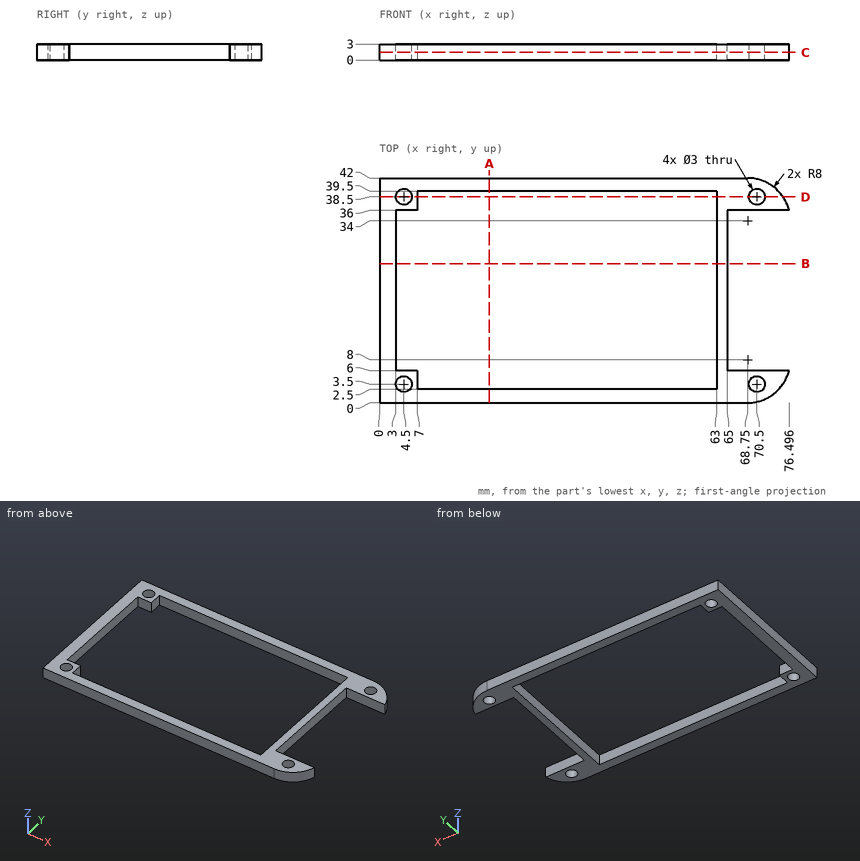
Could you check a few things on this drawing? It's one solid part, dimensions in mm from its lowest x, y, z. Round coordinates to 2 decimals unless told otherwise and drop trailing zeros. Order: outer loops, then holes, each group sorted by start corner. A loop starts at its lowest first (then second) coordinate and runs counter-clockwise, first axis right, second up. Notation, with made-up numbers: M -13,29 L -2,29 A29 ccw -2,56 Z; hole C -3,31 d9. An arc over 180 degrees is marked long. Return JSON: item names as keys, results as strings. Group by question number.
1. If we section it at C-C on z = 1.45: List the corners of the cut face in (x, y) for me, then the cut area to 3 significant figures.
2. Please list where these lines run through material, in increasing order: probe 1 along Y at (x, z) = (4.5, 1.7); probe 2 along Y at (x, z) = (70.5, 1.45); probe 3 along Y at (x, z) = (39, 1.5).
3. If we section it at A-A on x = 20.5: List the corners of the cut face in (y, z) for me.
4. If we section it at B-B on y = 26: List the corners of the cut face in (x, z) for me, then the cut area to 3 significant figures.
5. I'm going to push flat-ended pins straight in: pin 1 Ø4 at (x, y) = (70.5, 38.5) entering from +Z; pin 2 Ø0.9 at (y, z) = (5, 1.5) entering from +X; pin 3 Ø1.5 at (y, z) = (25, 2) entering from +X. Where does each tip first touch, or does it pass through?
6. If we section it at D-D on y = 38.5: List the corners of the cut face in (x, z) for me, then the cut area to 3 significant figures.
Reply:
{
 "1": {"outline": "M 0,0 L 68.75,0 A8 ccw 76.5,6 L 65,6 L 65,36 L 76.5,36 A8 ccw 68.75,42 L 0,42 Z; hole C 4.5,3.5 d3; hole M 3,6 L 7,6 L 7,2.5 L 63,2.5 L 63,39.5 L 7,39.5 L 7,36 L 3,36 Z; hole C 4.5,38.5 d3; hole C 70.5,3.5 d3; hole C 70.5,38.5 d3", "area": "624 mm^2"},
 "2": {"probe 1": "0 to 2, 5 to 6, 36 to 37, 40 to 42", "probe 2": "0.19 to 2, 5 to 6, 36 to 37, 40 to 41.81", "probe 3": "0 to 2.5, 39.5 to 42"},
 "3": {"outline": "M 0,0 L 2.5,0 L 2.5,3 L 0,3 Z; M 39.5,0 L 42,0 L 42,3 L 39.5,3 Z"},
 "4": {"outline": "M 0,0 L 3,0 L 3,3 L 0,3 Z; M 63,0 L 65,0 L 65,3 L 63,3 Z", "area": "15.0 mm^2"},
 "5": {"pin 1": "z = 3", "pin 2": "x = 76.33", "pin 3": "x = 65"},
 "6": {"outline": "M 0,0 L 3,0 L 3,3 L 0,3 Z; M 6,0 L 7,0 L 7,3 L 6,3 Z; M 63,0 L 69,0 L 69,3 L 63,3 Z; M 72,0 L 75.36,0 L 75.36,3 L 72,3 Z", "area": "40.1 mm^2"}
}
